```python
from build123d import *

# Parameters (mm, degrees)
BOSS_EXTRUDE1_DEPTH = 10
BOSS_EXTRUDE2_DEPTH = 80
SKETCH3_W           = 40
SKETCH3_H           = 10
BOSS_EXTRUDE3_DEPTH = 18.71
SKETCH4_W           = 10
SKETCH4_H           = 90
BOSS_EXTRUDE4_DEPTH = 50
CUT_EXTRUDE1_REACH  = 162.624
SKETCH6_R           = 3.5
CUT_EXTRUDE2_DEPTH  = 10
CUT_EXTRUDE3_DEPTH  = 10
SKETCH8_R           = 3
CUT_EXTRUDE4_DEPTH  = 10
SKETCH9_R           = 3
CUT_EXTRUDE5_DEPTH  = 10
SKETCH10_W          = 60
SKETCH10_H          = 10
BOSS_EXTRUDE5_DEPTH = 39
SKETCH11_R          = 11
CUT_EXTRUDE6_DEPTH  = 10
CUT_EXTRUDE7_START  = -10
CUT_EXTRUDE7_DEPTH  = 10
SKETCH13_R          = 10
BOSS_EXTRUDE6_DEPTH = 15
CUT_EXTRUDE8_START  = -8
SKETCH14_R          = 10
SKETCH14_R_2        = 7.5
CUT_EXTRUDE8_DEPTH  = 3
SKETCH15_R          = 10
BOSS_EXTRUDE7_DEPTH = 20
CUT_EXTRUDE9_START  = -8
SKETCH16_R          = 10
SKETCH16_R_2        = 7.5
CUT_EXTRUDE9_DEPTH  = 3


with BuildPart() as part:
    # Sketch1 → Boss-Extrude1 (new body)
    with BuildSketch(Plane(origin=(0, 0, 0), x_dir=(1, 0, 0), z_dir=(0, 1, 0))):
        Polygon((0, 0), (100, 0), (100, 40), (60, 40), (60, 80), (0, 80), align=None)
    extrude(amount=BOSS_EXTRUDE1_DEPTH)

    # Sketch2 → Boss-Extrude2 (add)
    with BuildSketch(Plane.XZ):
        Polygon((60, -40), (100, -40), (100, -30), (50, -30), (50, -80), (60, -80), align=None)
    extrude(amount=BOSS_EXTRUDE2_DEPTH)

    # Sketch3 → Boss-Extrude3 (add)
    with BuildSketch(Plane(origin=(0, 10, 0), x_dir=(1, 0, 0), z_dir=(0, 1, 0))):
        with Locations((80, 35)):
            Rectangle(SKETCH3_W, SKETCH3_H)
    extrude(amount=BOSS_EXTRUDE3_DEPTH)

    # Sketch4 → Boss-Extrude4 (add)
    with BuildSketch(Plane(origin=(0, 0, -80), x_dir=(-1, 0, 0), z_dir=(0, 0, -1))):
        with Locations((-55, -35)):
            Rectangle(SKETCH4_W, SKETCH4_H)
    extrude(amount=BOSS_EXTRUDE4_DEPTH)

    # Sketch5 → Cut-Extrude1 (cut, up to next)
    with BuildSketch(Plane.ZY.offset(-50), mode=Mode.PRIVATE) as cut_extrude1_sk1:
        Polygon((-80, -80), (-130, -30), (-130, -80), align=None)
    cut_extrude1_tool1 = extrude(cut_extrude1_sk1.sketch, amount=-CUT_EXTRUDE1_REACH, mode=Mode.PRIVATE) & part.part
    add(cut_extrude1_tool1.solids().sort_by_distance((50, -63.333333, -113.333333))[0], mode=Mode.SUBTRACT)

    # Sketch6 → Cut-Extrude2 (cut)
    with BuildSketch(Plane(origin=(0, 10, 0), x_dir=(1, 0, 0), z_dir=(0, 1, 0))):
        with Locations(Location((7, 50, 0), (0, 0, 270))):
            Circle(SKETCH6_R)
        with Locations(Location((53, 50, 0), (0, 0, 270))):
            Circle(SKETCH6_R)
    extrude(amount=-CUT_EXTRUDE2_DEPTH, mode=Mode.SUBTRACT)

    # Sketch7 → Cut-Extrude3 (cut)
    with BuildSketch(Plane.ZY.offset(-50)):
        Polygon((-50, 0), (-43, 0), (-43, -6), (-57, -6), (-57, 0), align=None)
    extrude(amount=-CUT_EXTRUDE3_DEPTH, mode=Mode.SUBTRACT)

    # Sketch8 → Cut-Extrude4 (cut)
    with BuildSketch(Plane.XY.offset(-30)):
        with Locations((70, 18.71)):
            Circle(SKETCH8_R)
        with Locations((90, 18.71)):
            Circle(SKETCH8_R)
        with Locations((70, -15)):
            Circle(SKETCH8_R)
        with Locations((90, -15)):
            Circle(SKETCH8_R)
        with Locations((90, -65)):
            Circle(SKETCH8_R)
        with Locations((70, -65)):
            Circle(SKETCH8_R)
    extrude(amount=-CUT_EXTRUDE4_DEPTH, mode=Mode.SUBTRACT)

    # Sketch9 → Cut-Extrude5 (cut)
    with BuildSketch(Plane.ZY.offset(-50)):
        with Locations((-50, -15)):
            Circle(SKETCH9_R)
        with Locations((-70, -15)):
            Circle(SKETCH9_R)
        with Locations((-70, -65)):
            Circle(SKETCH9_R)
        with Locations((-50, -65)):
            Circle(SKETCH9_R)
        with Locations((-90, -1.3)):
            Circle(SKETCH9_R)
        with Locations((-120, -1.3)):
            Circle(SKETCH9_R)
        with Locations((-90, -21.3)):
            Circle(SKETCH9_R)
        with Locations((-120, -21.3)):
            Circle(SKETCH9_R)
    extrude(amount=-CUT_EXTRUDE5_DEPTH, mode=Mode.SUBTRACT)

    # Sketch10 → Boss-Extrude5 (add)
    with BuildSketch(Plane(origin=(0, 10, 0), x_dir=(1, 0, 0), z_dir=(0, 1, 0))):
        with Locations((30, 35)):
            Rectangle(SKETCH10_W, SKETCH10_H)
        with Locations((30, 65)):
            Rectangle(SKETCH10_W, SKETCH10_H)
    extrude(amount=BOSS_EXTRUDE5_DEPTH)

    # Sketch11 → Cut-Extrude6 (cut)
    with BuildSketch(Plane.XY.offset(-30)):
        with Locations((30, 32)):
            Circle(SKETCH11_R)
    extrude(amount=-CUT_EXTRUDE6_DEPTH, mode=Mode.SUBTRACT)

    # Sketch12 → Cut-Extrude7 (cut)
    with BuildSketch(Plane(origin=(0, 0, -70), x_dir=(-1, 0, 0), z_dir=(0, 0, -1)).offset(CUT_EXTRUDE7_START)):
        with BuildLine():
            Line((-19, 49), (-19, 32))
            ThreePointArc((-19, 32), (-30, 21), (-41, 32))
            Line((-41, 32), (-41, 49))
            Line((-41, 49), (-19, 49))
        make_face()
    extrude(amount=CUT_EXTRUDE7_DEPTH, mode=Mode.SUBTRACT)

    # Sketch13 → Boss-Extrude6 (add)
    with BuildSketch(Plane.XY.offset(-30)):
        with Locations(Location((65, -40, 0), (0, 0, 180))):
            Circle(SKETCH13_R)
    extrude(amount=BOSS_EXTRUDE6_DEPTH)

    # Sketch14 → Cut-Extrude8 (cut)
    with BuildSketch(Plane.XY.offset(-15).offset(CUT_EXTRUDE8_START)):
        with Locations(Location((65, -40, 0), (0, 0, 180))):
            Circle(SKETCH14_R)
        with Locations((65, -40)):
            Circle(SKETCH14_R_2, mode=Mode.SUBTRACT)
    extrude(amount=CUT_EXTRUDE8_DEPTH, mode=Mode.SUBTRACT)

    # Sketch15 → Boss-Extrude7 (add)
    with BuildSketch(Plane.ZY.offset(-50)):
        with Locations(Location((-45, -40, 0), (0, 0, 180))):
            Circle(SKETCH15_R)
    extrude(amount=BOSS_EXTRUDE7_DEPTH)

    # Sketch16 → Cut-Extrude9 (cut)
    with BuildSketch(Plane.ZY.offset(-30).offset(CUT_EXTRUDE9_START)):
        with Locations(Location((-45, -40, 0), (0, 0, 180))):
            Circle(SKETCH16_R)
        with Locations((-45, -40)):
            Circle(SKETCH16_R_2, mode=Mode.SUBTRACT)
    extrude(amount=CUT_EXTRUDE9_DEPTH, mode=Mode.SUBTRACT)


solid = part.part
```
CAD build for the part. Positions are in the model's coordinates, mm. A direction names the side the tool comes from. Round coordinates to 2 decimals unless told otherwise and drop trailing zeros. Order: outer loops, then holes, each group sorted by start corner. A loop starts at its lowest first (then second) coordinate and runs counter-clockwise, first axis right, second up.
Item 1: Mould opens along X. For faces 5 (the face through (100, -22, -32)), 6 (the face through (55, -10, -130)), 7 (the face through (73, -34, -27)), 8 (the face through (40.161, 27.787, -34.93)) say: pulls with the +X half, pulls with the -X half, needs draft (parallel to the pull), parting line crosses it, or undercut.
Item 2: Probe line 1 along X through (y, z) = (6, -50); line 2 along Z through (x, y) = (57, -1); line 3 along Y through (x, z) = (90, -33). List the from-to ranges inside material, lowest first.
Item 3: Saw through at D-D on x = 53. State how many separate pieces and enclosed holes the cut face has, then the cut area to 3 significant figures.
Item 4: Tool access for faces 1 (the face through (30, 10, -50)), 2 (the face through (60, 39, -35)), 3 (the face through (55, -6, -50)), 4 (the face through (43.8, 10, -79.6)): list every direction of +Z, -Z, +X, -X, +Y, -Y with a clear straight run to the whole face (end or side of a thin tool).
Item 5: Saw through at B-B on y = -21.3. Write the cut outline in (x, z), then the cut area to 3 significant figures.
Item 6: Saw through at A-A on z = -90. Write the cut outline in (x, y).
Item 7: Pin check, flat tips, straight feed: pin 1 (2 mm diameter, centred on y = -17.5, z = -88, fed in from +X); pin 2 (9.5 mm diameter, centred on x = 70, y = 18.71, fed in from +Z); pin 3 (2 mm diameter, centred on x = 31.5, z = -71.5, fed in from -Y). Stop position of each tip, or through.
Item 8: Saw through at C-C on x = 23.5. Write the cut outline in (y, z), then the cut area to 3 significant figures.
Reported:
1. face 5: pulls with the +X half
1. face 6: needs draft
1. face 7: parting line crosses it
1. face 8: undercut
2. line 1: x = 0 to 3.5, 10.5 to 49.5, 56.5 to 60
2. line 2: z = -130 to -122.98, -117.02 to -92.98, -87.02 to -57, -43 to -30
2. line 3: y = -80 to -68, -62 to -18, -12 to 15.71, 21.71 to 28.71
3. separate pieces: 1
3. enclosed holes: 8
3. area: 8,450 mm2
4. face 1: +X, -X, +Y
4. face 2: +Z, -Z, +X, +Y
4. face 3: +X, -X
4. face 4: -Z, +X, -X, +Y
5. outline: (50, -130) - (60, -130) - (60, -123) - (50, -123) - close; (50, -117) - (60, -117) - (60, -93) - (50, -93) - close; (50, -87) - (60, -87) - (60, -40) - (100, -40) - (100, -30) - (50, -30) - close
5. area: 1,280 mm2
6. outline: (50, -70) - (60, -70) - (60, -24.3) - (50, -24.3) - close; (50, -18.3) - (60, -18.3) - (60, -4.3) - (50, -4.3) - close; (50, 1.7) - (60, 1.7) - (60, 10) - (50, 10) - close
7. pin 1: stops at x = 60
7. pin 2: stops at z = -30
7. pin 3: stops at y = 0
8. outline: (0, -80) - (10, -80) - (10, -70) - (23.13, -70) - (23.13, -60) - (10, -60) - (10, -40) - (23.13, -40) - (23.13, -30) - (10, -30) - (10, 0) - (0, 0) - close; (40.87, -40) - (49, -40) - (49, -30) - (40.87, -30) - close
8. area: 1,140 mm2
